```python
from build123d import *

# Parameters (mm, degrees)
EXTRUDE_1_DEPTH = 120
CHAMFER_2_SIZE  = 0.4


with BuildPart() as part:
    # 草图1 → 凸台-拉伸1 (new body)
    with BuildSketch(Plane(origin=(0, 0, 0), x_dir=(1, 0, 0), z_dir=(0, 1, 0))):
        with BuildLine():
            Line((-24.5, 0), (-16.5, 0))
            ThreePointArc((-16.5, 0), (0, 16.5), (16.5, 0))
            Line((16.5, 0), (24.5, 0))
            ThreePointArc((24.5, 0), (0, 24.5), (-24.5, 0))
        make_face()
    extrude(amount=EXTRUDE_1_DEPTH)

    # 倒角1
    # the kernel refuses this chamfer: 0.4 mm, written as the material it takes off along each edge
    with BuildSketch(Plane(origin=(15.471326805, 120, 0), x_dir=(0, -0.9996219169112966, 0.027495876610585543), z_dir=(1, 0, 0)), Plane(origin=(-25.528673195, 120, 0), x_dir=(0, -0.9996219169112966, 0.027495876610585543), z_dir=(1, 0, 0))) as chamfer_1_piece_1:
        with BuildLine():
            Line((0.411469278, 0), (-0.022618862, 0.410847117))
            Line((-0.022618862, 0.410847117), (-0.030615837, 0.41062715))
            ThreePointArc((-0.030615837, 0.41062715), (-0.013651691, 0.205359132), (-0.007996975, -0.000219967))
            Line((-0.007996975, -0.000219967), (0.000219967, -0.007996975))
            ThreePointArc((0.000219967, -0.007996975), (0.205799066, -0.00234226), (0.411689245, -0.007996975))
            Line((0.411689245, -0.007996975), (0.411469278, 0))
        make_face()
    extrude(amount=10.05734639, mode=Mode.SUBTRACT)
    with BuildSketch(Plane(origin=(15.471326805, 0, 0), x_dir=(0, 0.9996219169112968, 0.02749587661058639), z_dir=(1, 0, 0)), Plane(origin=(-25.528673195, 0, 0), x_dir=(0, 0.9996219169112968, 0.02749587661058639), z_dir=(1, 0, 0))) as chamfer_1_piece_2:
        with BuildLine():
            Line((0.411469278, 0), (-0.022618862, -0.410847117))
            Line((-0.022618862, -0.410847117), (-0.030615837, -0.41062715))
            ThreePointArc((-0.030615837, -0.41062715), (-0.013651691, -0.205359132), (-0.007996975, 0.000219967))
            Line((-0.007996975, 0.000219967), (0.000219967, 0.007996975))
            ThreePointArc((0.000219967, 0.007996975), (0.205799066, 0.00234226), (0.411689245, 0.007996975))
            Line((0.411689245, 0.007996975), (0.411469278, 0))
        make_face()
    extrude(amount=10.05734639, mode=Mode.SUBTRACT)
    with BuildSketch(Plane(origin=(24.5, -1.045299528, 0), x_dir=(-0.9996215998180249, 0, 0.0275074022265361), z_dir=(0, 1, 0))) as chamfer_1_piece_3:
        with BuildLine():
            Line((0.414696078, 0), (-0.019340993, -0.417672243))
            Line((-0.019340993, -0.417672243), (-0.027340517, -0.417584944))
            ThreePointArc((-0.027340517, -0.417584944), (-0.012856137, -0.208775648), (-0.007996973, 0.000220059))
            Line((-0.007996973, 0.000220059), (0.000220059, 0.007996973))
            ThreePointArc((0.000220059, 0.007996973), (0.207411207, 0.002295525), (0.414916137, 0.007996973))
            Line((0.414916137, 0.007996973), (0.414696078, 0))
        make_face()
    extrude(amount=122.090599055, mode=Mode.SUBTRACT)
    with BuildSketch(Plane(origin=(16.5, -1.017165076, 0), x_dir=(-0.039969745571149635, 0, -0.9992008904314376), z_dir=(0, 1, 0))) as chamfer_1_piece_4:
        with BuildLine():
            Line((0.402032829, 0), (-0.027426276, -0.405940594))
            Line((-0.027426276, -0.405940594), (-0.035419883, -0.405620836))
            ThreePointArc((-0.035419883, -0.405620836), (-0.016121703, -0.20287395), (-0.007993607, 0.000319758))
            Line((-0.007993607, 0.000319758), (0.000319758, 0.007993607))
            ThreePointArc((0.000319758, 0.007993607), (0.201049453, 0.001188032), (0.4021633, 0.007998936))
            Line((0.4021633, 0.007998936), (0.402032829, 0))
        make_face()
    extrude(amount=122.034330152, mode=Mode.SUBTRACT)
    with BuildSketch(Plane(origin=(-16.5, -1.017165076, 0), x_dir=(-0.9996224657663016, 0, 0.02747591554978717), z_dir=(0, 1, 0))) as chamfer_1_piece_5:
        with BuildLine():
            Line((0.40686603, 0), (-0.027100476, -0.401118387))
            Line((-0.027100476, -0.401118387), (-0.035090013, -0.400709363))
            ThreePointArc((-0.035090013, -0.400709363), (-0.014737795, -0.200512073), (-0.00799698, 0.000219807))
            Line((-0.00799698, 0.000219807), (0.000219807, 0.00799698))
            ThreePointArc((0.000219807, 0.00799698), (0.203499246, 0.002409582), (0.407085838, 0.00799698))
            Line((0.407085838, 0.00799698), (0.40686603, 0))
        make_face()
    extrude(amount=122.034330152, mode=Mode.SUBTRACT)
    with BuildSketch(Plane(origin=(-24.5, -1.045299528, 0), x_dir=(0.9996215998180249, 0, 0.02750740222653502), z_dir=(0, 1, 0))) as chamfer_1_piece_6:
        with BuildLine():
            Line((0.414696078, 0), (-0.019340993, 0.417672243))
            Line((-0.019340993, 0.417672243), (-0.027340517, 0.417584944))
            ThreePointArc((-0.027340517, 0.417584944), (-0.012856137, 0.208775648), (-0.007996973, -0.000220059))
            Line((-0.007996973, -0.000220059), (0.000220059, -0.007996973))
            ThreePointArc((0.000220059, -0.007996973), (0.207411207, -0.002295525), (0.414916137, -0.007996973))
            Line((0.414916137, -0.007996973), (0.414696078, 0))
        make_face()
    extrude(amount=122.090599055, mode=Mode.SUBTRACT)

    # 倒角2
    chamfer_2_edges = [part.edges().sort_by_distance(p)[0] for p in [
        (0, 0, -24.5),
        (0, 0, -16.5),
        (0, 120, -16.5),
        (0, 120, -24.5),
    ]]
    chamfer(chamfer_2_edges, length=CHAMFER_2_SIZE)


solid = part.part
```
CAD build for the part. Positions are in the model's coordinates, mm. Round coordinates to 2 decimals unless told otherwise and drop trailing zeros. Write each loop counter-clockwise with the first axis right and the second up, starting at its lowest first coordinate (ties: lowest second). Pieces come first, ordered by that corner, then holes.
Item 1: Mould opens along X. For faces 1 (the cylindrical face through (-0.357, 59.166, -16.496)), 2 (the flat face through (-21, 59, 0)), 3 (the conical face through (-0.363, 119.714, -16.61)), 4 (the conical face through (0.53, 0.114, -24.208)) say: released by +X, released by -X, zero draft, split by the parting line, or undercut.
Filled in:
face 1: undercut
face 2: zero draft
face 3: undercut
face 4: split by the parting line
Item 2: Band-saw the part on A-A on x = 0. Write the cut outline in (y, z), then the cut area to 3 significant figures.
Filled in:
outline: (0, -24.1) - (0.4, -24.5) - (119.6, -24.5) - (120, -24.1) - (120, -16.9) - (119.6, -16.5) - (0.4, -16.5) - (0, -16.9) - close
area: 960 mm2
Item 3: Drop flat-ended pins along their axis: pin 1 Ø1 at (y, z) = (49, -9) entering from -X; pin 2 Ø12 at (y, z) = (96, -3) entering from -X; pin 3 Ø2 at (x, y) = (-3, 48.5) entering from +Z; pin 4 Ø1 at (y, z) = (34.5, -7.5) entering from +X. Give the stop position or say it passes through.
Filled in:
pin 1: stops at x = -22.98
pin 2: stops at x = -24.5
pin 3: stops at z = -16.01
pin 4: stops at x = 23.48
Item 4: Drill centre lines: L1, parallel to X at y = 20, z = -9; L2, parallel to X at y = 102.5, z = -8.5; L3, parallel to Z at x = -12.5, y = 58. Where is each one in solid material? Low to high.
Filled in:
L1: x = -22.79 to -13.83, 13.83 to 22.79
L2: x = -22.98 to -14.14, 14.14 to 22.98
L3: z = -21.07 to -10.77
